CAD build for the part. Positions are in the model's coordinates, mm. Face numbers are marked on the shaded views. A direction names the side the tool comes from. Coordinates: 2 decimals unless noted, no trailing zeros. Loops run counter-clockwise (first coordinate to the right, second up) from the corner with the lowest first, then second, coordinate; pieces in that order, holes last. Notation, with made-up numbers: (30.5, 2.25) -> (76.5, 2.25) arc R17 ccw to (76.5, 31.25) -> close; hole circle Ø4 at (-9, 60). An arc over 180 degrees is marked (long way). Write item = value, one per line. Start each with the question number.
(1) Band-saw the part on A-A (y = 16). Write the cut outline in (x, z).
(2) Tool access for the marked faces 4 and 5: list every direction of +Z, -Z, +X, -X, +Y, -Y with a clear straight run to the whole face (end or side of a thin tool).
(3) Pull direction X, two halves, no side cores. Call the marked faces 1, 2 and 3: +X half, -X half, draft (parallel to the pull), parting line (faces both ways), or undercut.
(4) Drill centre lines: line 1 (Z direction, x = -0.75, y = 4.5); line 2 (X direction, y = 13.75, z = 4.25); line 3 (Y direction, x = -7.5, z = 4.25). Where is each one in solid material? Low to high. Write a range as from..to.
```python
from build123d import *

# Parameters (mm, degrees)
SKETCH1_W           = 16.2
SKETCH1_H           = 12.1
BOSS_EXTRUDE1_DEPTH = 20
SKETCH2_W           = 14.2
SKETCH2_H           = 10.1
SKETCH2_2_W         = 14.2
SKETCH2_2_H         = 10.1
CUT_EXTRUDE1_DEPTH  = 22.5


with BuildPart() as part:
    # Sketch1 → Boss-Extrude1 (new body)
    with BuildSketch(Plane(origin=(0, 0, 0), x_dir=(1, 0, 0), z_dir=(0, 1, 0))):
        Rectangle(SKETCH1_W, SKETCH1_H)
    extrude(amount=BOSS_EXTRUDE1_DEPTH)

    # Sketch2 → section 1 of loft1
    with BuildSketch(Plane(origin=(0, 21.5, 0), x_dir=(1, 0, 0), z_dir=(0, 1, 0)), mode=Mode.PRIVATE) as loft1_s1:
        Rectangle(SKETCH2_W, SKETCH2_H)
    # loft from a face of the part (loft1)
    loft([part.faces().sort_by_distance((0, 20, 0))[0], loft1_s1.sketch])

    # Sketch2_2 → Cut-Extrude1 (cut, through all)
    with BuildSketch(Plane(origin=(0, 21.5, 0), x_dir=(1, 0, 0), z_dir=(0, 1, 0))):
        Rectangle(SKETCH2_2_W, SKETCH2_2_H)
    extrude(amount=-CUT_EXTRUDE1_DEPTH, mode=Mode.SUBTRACT)


solid = part.part
```
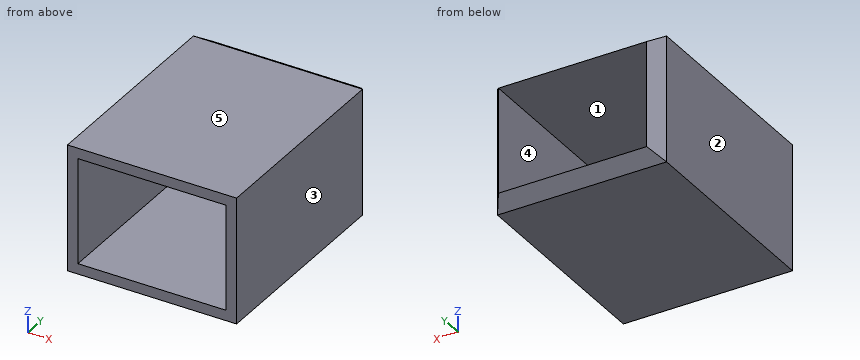
Findings below:
q1.outline = (-8.1, -6.05) -> (8.1, -6.05) -> (8.1, 6.05) -> (-8.1, 6.05) -> close; hole (-7.1, -5.05) -> (7.1, -5.05) -> (7.1, 5.05) -> (-7.1, 5.05) -> close
q2.face_4 = +Y, -Y
q2.face_5 = +Z, +X, -X, +Y, -Y
q3.face_1 = undercut
q3.face_2 = -X half
q3.face_3 = +X half
q4.line_1 = -6.05..-5.05, 5.05..6.05
q4.line_2 = -8.1..-7.1, 7.1..8.1
q4.line_3 = 0..20.9
